Autodesk Inventor part; units mm, degrees
ref_plane "YZ Plane" through (0, 0, 0) normal (1, 0, 0) x (0, 1, 0)
ref_plane "XZ Plane" through (0, 0, 0) normal (0, 1, 0) x (-1, 0, 0)
ref_plane "XY Plane" through (0, 0, 0) normal (0, 0, 1) x (1, 0, 0)
sketch "Sketch1" plane through (0, 0, 0) normal (0, 0, 1) x (1, 0, 0)
  line L0 (0, 0) -> (44, 0)
  line L1 (44, 0) -> (44, 44)
  line L2 (44, 44) -> (0, 44)
  line L3 (0, 44) -> (0, 0)
  dimension "d0" = 44
  dimension "d1" = 44
extrude "Extrusion1" add sketch "Sketch1" along normal blind 4
chamfer "Chamfer1" distance 4 angle 45 4 edges at (22, 44, 4) (44, 22, 4) (22, 0, 4) (0, 22, 4)
sketch "Sketch2" plane through (0, 0, 4) normal (0, 0, 1) x (1, 0, 0)
  line L0 (40, 4) -> (4, 4)
  line L1 (40, 40) -> (40, 4)
  line L2 (4, 40) -> (40, 40)
  line L3 (4, 4) -> (4, 40)
  line L4 (4, 40) -> (40, 40)
  line L5 (4, 40) -> (5, 40)
  line L6 (5, 40) -> (5, 39)
  line L7 (5, 39) -> (39, 39)
  line L8 (39, 39) -> (39, 5)
  line L9 (39, 5) -> (5, 5)
  line L10 (5, 5) -> (5, 39)
  line L11 (5, 39) -> (7, 39)
  line L12 (7, 39) -> (7, 37)
  line L13 (7, 37) -> (37, 37)
  line L14 (37, 37) -> (37, 7)
  line L15 (37, 7) -> (7, 7)
  line L16 (7, 7) -> (7, 37)
  point P0 (0, 0)
  dimension "d7" = 1
  dimension "d8" = 1
  dimension "d9" = 34
  dimension "d10" = 34
  dimension "d11" = 2
  dimension "d12" = 2
  dimension "d13" = 30
  dimension "d14" = 30
extrude "Extrusion2" cut sketch "Sketch2" against normal blind 2 contours L7 L8 L9 L10
chamfer "Chamfer2" distance 1 angle 45 8 edges at (22, 37, 2) (22, 39, 2) (5, 22, 2) (22, 7, 2) (7, 22, 2) (22, 5, 2) (37, 22, 2) (39, 22, 2)
properties part number "clear-square-notched"
Verification items for the finished model (mm, model axes). A direction names the side the tool comes from. Coordinates: 2 decimals unless noted, no trailing zeros. Put each result on its own line as item: value. Start each with the question number.
1. Mould release check, pull along Y, two halves, no side actions. Record for faces 3 (the flat face through (20.6, 4.8, 4)), 4 (the flat face through (22, 2, 2)), 5 (the flat face through (37, 22.2, 3.5)): released by +Y, released by -Y, zero draft, split by the parting line, or undercut.
2. Material ranges on L1, parallel to Y at x = 20.5, z = 3; L2, parallel to Y at x = 29, z = 2.5; L3, parallel to X at y = 36.5, z = 2.7, recorded low to high. Write a range as [from, to].
3. Go/stop test with flat-tipped pins: pin 1 Ø1.1 at (x, z) = (23, 3.5) entering from +Y; pin 2 Ø0.8 at (y, z) = (28.5, 3.5) entering from -X; pin 3 Ø0.5 at (y, z) = (17.5, 3.5) entering from +X. Record where each tip stops, or that it passes through.
4. Access from +Z, -Z, +X, -X, +Y, -Y to the whole of each face (thin tool, end or side, straight path). Record for faces 1 (the flat face through (5, 21.8, 3.5)), 2 (the flat face through (22, 22, 4)).
Computed:
1. face 3: zero draft
1. face 4: released by -Y
1. face 5: undercut
2. L1: [3, 5], [7, 37], [39, 41]
2. L2: [2.5, 5.5], [6.5, 37.5], [38.5, 41.5]
2. L3: [2.7, 5.3], [6.7, 37.3], [38.7, 41.3]
3. pin 1: y = 41.05
3. pin 2: x = 3.1
3. pin 3: x = 40.75
4. face 1: +Z
4. face 2: +Z, +X, -X, +Y, -Y
